Can you work these out from the model? Positions are in its coordinate system, mm. A direction names the side the tool comes from. Round coordinates to 2 decimals unless told otherwise and drop trailing zeros. Order: outer loops, then holes, each group sorted by start corner. A loop starts at its lowest first (then second) coordinate and runs counter-clockwise, first axis right, second up. Notation, with made-up numbers: (43.5, -40) -> (71.5, -40) arc R29 cw to (71.5, -18) -> close; hole circle Ø10 at (-1, 5.25). An arc over 180 degrees is marked (long way). One line per item, written item: value.
```python
from build123d import *

# Parameters (mm, degrees)
F2_T     = 1.2
F4_D     = 300
F4_DEPTH = 1.201


with BuildPart() as f1:
    # F0 (on Front) → F1 (revolve)
    with BuildSketch(Plane.XZ):
        Polygon((-3.6914059892, 36.4218764007), (-35.1914092898, 0), (0, 0), (0, 63.2460936904), (-3.6914059892, 63.2460936904), align=None)
    revolve(axis=Axis((0, 0, 31.6230468452), (0, 0, -1)))

    # F2 (hollow, outwards: the wall grows on the outside; the body as it was is the cavity)
    f2_inside = f1.part
    offset(amount=F2_T, kind=Kind.INTERSECTION)
    add(f2_inside, mode=Mode.SUBTRACT)

    # F4 (through all, one way)
    with BuildSketch(Plane.XY):
        with Locations((0, 0)):
            Circle(F4_D / 2)
    extrude(amount=-F4_DEPTH, mode=Mode.SUBTRACT)


solid = f1.part
```
Q1. I want a section at D-D on z = 12. List the corners of the cut face in (x, y) for me.
Answers below:
outline: circle Ø52.8 at (0, 0); hole circle Ø49.63 at (0, 0)
Q2. On a 3-axis mill with a long thin cutter (end or side, diameter ignored), from which of +Z, -Z, +X, -X, +Y, -Y can I reach the whole of each face in a straight line? I mean faces 5 (the face through (3.688, 0.162, 49.646)), 6 (the face through (3.88, -2.98, 50.46)), 7 (the face through (30, -19, 0)). Say none if no direction works.
Answers below:
face 5: -Z
face 6: +Z
face 7: -Z, +X, -X, +Y, -Y
Q3. Please list where these lines run through material, in increasing order: line 1 along Y through (x, z) = (0, 53.75); line 2 along Y through (x, z) = (1, 55); line 3 along X through (y, z) = (4, 33).
Answers below:
line 1: -4.89 to -3.69, 3.69 to 4.89
line 2: -4.79 to -3.55, 3.55 to 4.79
line 3: -7.2 to -5.31, 5.31 to 7.2
Q4. We'd pull the mould along Y, two halves only. Please class faces 1 (the face through (10.05, -7.7, 26.05)), 2 (the face through (0, 0, 64.446)), 3 (the face through (2.26, -10.18, 30.47)), 4 (the face through (0, 0, 63.246)): released by +Y, released by -Y, zero draft, split by the parting line, or undercut.
Answers below:
face 1: undercut
face 2: zero draft
face 3: split by the parting line
face 4: undercut
Q5. I want a section at A-A on y = 0. List the corners of the cut face in (x, z) for me, plus the area to 3 significant figures.
Answers below:
outline: (-36.78, 0) -> (-35.19, 0) -> (-3.69, 36.42) -> (-3.69, 63.25) -> (3.69, 63.25) -> (3.69, 36.42) -> (35.19, 0) -> (36.78, 0) -> (4.89, 36.87) -> (4.89, 64.45) -> (-4.89, 64.45) -> (-4.89, 36.87) -> close
area: 192 mm^2
Q6. Will these pins go through, and if not, where does the flat tip stop? pin 1 Ø6 at (y, z) = (21, 8.5) entering from -X; pin 2 Ø2 at (y, z) = (-5.5, 16.5) entering from +X; pin 3 Ø3 at (x, y) = (21.5, 20) entering from -Z.
Answers below:
pin 1: x = -24.98
pin 2: x = 22.75
pin 3: z = 5
Q7. I want a section at C-C on z = 19. List the corners of the cut face in (x, y) for me.
Answers below:
outline: circle Ø40.69 at (0, 0); hole circle Ø37.52 at (0, 0)
